CAD build for the part. Positions are in the model's coordinates, mm. A direction names the side the tool comes from. Coordinates: 2 decimals unless noted, no trailing zeros. Loops run counter-clockwise (first coordinate to the right, second up) from the corner with the lowest first, then second, coordinate; pieces in that order, holes last. Notation, with made-up numbers: (-28, 19.25) -> (21, 19.25) arc R11 ccw to (21, 29.25) -> close; hole circle Ø4 at (1, 1.5). An arc over 180 degrees is marked (long way). Write item = value, one per line. Start each with the question number.
(1) Flat gauge pins, fed straight in: P1, Ø12.5, axis at x = -0.5, z = 35.5, coming from the -Y side; P2, Ø4, axis at x = 7.5, y = -12, coming from the +Z side; P3, Ø6, axis at x = -1.5, y = -17.5, coming from the +Z side. Where does each tip first touch, or does it go through?
(2) Drill centre lines: line 1 (Z direction, x = -10, y = -19.5); line 2 (Y direction, x = -4.25, z = 6); line 3 (Y direction, x = -2.25, z = 31.5). Where is each one in solid material? Low to high. Write a range as from..to.
(3) Band-saw the part on D-D (x = 4.5). Write the cut outline in (y, z), and give its area (3 significant figures).
(4) Band-saw the part on A-A (x = 0). Write the cut outline in (y, z) (3 decimals), and give its area (3 significant figures).
(5) Pull direction Y, two halves, no side cores. Call faces 6 (the face through (0, -5, -30.48)), 7 (the face through (3, 10.16, 10)), 8 (the face through (-2.06, 2.5, 3.4)), 9 (the face through (4, 5.08, 36)): +Y half, -Y half, draft (parallel to the pull), parting line (faces both ways), or undercut.
(6) Band-saw the part on B-B (z = 35.56). Write the cut outline in (x, y) (3 decimals).
(7) Tool access for faces 1 (the face through (1.5, 7.6, 9.9)), 2 (the face through (-2.06, 2.5, 26.26)), 3 (the face through (4, 5.08, 13)), 4 (the face through (0.178, -38.939, 17.173)), 5 (the face through (12.7, 0, -11)): list every direction of +Z, -Z, +X, -X, +Y, -Y with a clear straight run to the whole face (end or side of a thin tool).
(8) Band-saw the part on C-C (y = 1). Write the cut outline in (x, z) (3 decimals), and give its area (3 significant figures).
```python
from build123d import *

# Parameters (mm, degrees)
F1_DEPTH = 12.7
F2_R     = 3.175
F3_DEPTH = 10.161
F2_R_2   = 9.525
F4_DEPTH = 5.08


with BuildPart() as f1:
    # F0 (on Right) → F1 (new body, symmetric)
    with BuildSketch(Plane.YZ):
        with BuildLine():
            Line((0, 50.8), (0, 0))
            ThreePointArc((0, 0), (-20.32, -20.32), (-40.64, 0))
            ThreePointArc((-40.64, 0), (-39.246403, 7.395517), (-35.256765, 13.776627))
            Line((-35.256765, 13.776627), (-42.725147, 20.664941))
            ThreePointArc((-42.725147, 20.664941), (-48.709604, 11.093275), (-50.8, 0))
            ThreePointArc((-50.8, 0), (-41.872615, -21.552615), (-20.32, -30.48))
            ThreePointArc((-20.32, -30.48), (1.232615, -21.552615), (10.16, 0))
            Line((10.16, 0), (10.16, 50.8))
            Line((10.16, 50.8), (0, 50.8))
        make_face()
        with BuildLine():
            Line((10.16, -30.48), (10.16, 0))
            ThreePointArc((10.16, 0), (1.232615, -21.552615), (-20.32, -30.48))
            Line((-20.32, -30.48), (10.16, -30.48))
        make_face()
    extrude(amount=F1_DEPTH, both=True)

    # F2 (on face) → F3 (cut, through all)
    with BuildSketch(Plane.XZ):
        with Locations((0, 35.56)):
            Circle(F2_R)
        with Locations((0, 12.7)):
            Circle(F2_R)
    extrude(amount=-F3_DEPTH, mode=Mode.SUBTRACT)

    # F2 (on face) → F4 (cut)
    with BuildSketch(Plane.XZ):
        with Locations((0, 35.56)):
            Circle(F2_R_2)
        with Locations((0, 35.56)):
            Circle(F2_R, mode=Mode.SUBTRACT)
        with Locations((0, 12.7)):
            Circle(F2_R_2)
        with Locations((0, 12.7)):
            Circle(F2_R, mode=Mode.SUBTRACT)
    extrude(amount=-F4_DEPTH, mode=Mode.SUBTRACT)


solid = f1.part
```
Findings below:
q1.P1 = 5.08
q1.P2 = -17.5
q1.P3 = -19.47
q2.line_1 = -30.48..-20.3
q2.line_2 = -50.2..-39.73, 5.08..10.16
q2.line_3 = 5.08..10.16
q3.outline = (-50.8, 0) arc R30.48 ccw to (-20.32, -30.48) -> (10.16, -30.48) -> (10.16, 50.8) -> (0, 50.8) -> (0, 43.95) -> (5.08, 43.95) -> (5.08, 27.17) -> (0, 27.17) -> (0, 21.09) -> (5.08, 21.09) -> (5.08, 4.31) -> (0, 4.31) -> (0, 0) arc R20.32 cw (long way) to (-35.26, 13.78) -> (-42.73, 20.66) arc R30.48 ccw to start
q3.area = 1,550 mm²
q4.outline = (-50.8, 0) arc R30.48 ccw to (-20.32, -30.48) -> (10.16, -30.48) -> (10.16, 9.525) -> (5.08, 9.525) -> (5.08, 3.175) -> (0, 3.175) -> (0, 0) arc R20.32 cw (long way) to (-35.257, 13.777) -> (-42.725, 20.665) arc R30.48 ccw to start; (0, 22.225) -> (5.08, 22.225) -> (5.08, 15.875) -> (10.16, 15.875) -> (10.16, 32.385) -> (5.08, 32.385) -> (5.08, 26.035) -> (0, 26.035) -> close; (0, 45.085) -> (5.08, 45.085) -> (5.08, 38.735) -> (10.16, 38.735) -> (10.16, 50.8) -> (0, 50.8) -> close
q4.area = 1,460 mm²
q5.face_6 = draft
q5.face_7 = +Y half
q5.face_8 = undercut
q5.face_9 = -Y half
q6.outline = (-12.7, 0) -> (-9.525, 0) -> (-9.525, 5.08) -> (-3.175, 5.08) -> (-3.175, 10.16) -> (-12.7, 10.16) -> close; (3.175, 5.08) -> (9.525, 5.08) -> (9.525, 0) -> (12.7, 0) -> (12.7, 10.16) -> (3.175, 10.16) -> close
q7.face_1 = +Y
q7.face_2 = -Y
q7.face_3 = none
q7.face_4 = +Z, +X, -X
q7.face_5 = +Z, -Z, +X, +Y, -Y
q8.outline = (-12.7, -30.48) -> (12.7, -30.48) -> (12.7, 50.8) -> (-12.7, 50.8) -> close; hole circle Ø19.05 at (0, 12.7); hole circle Ø19.05 at (0, 35.56)
q8.area = 1,490 mm²
